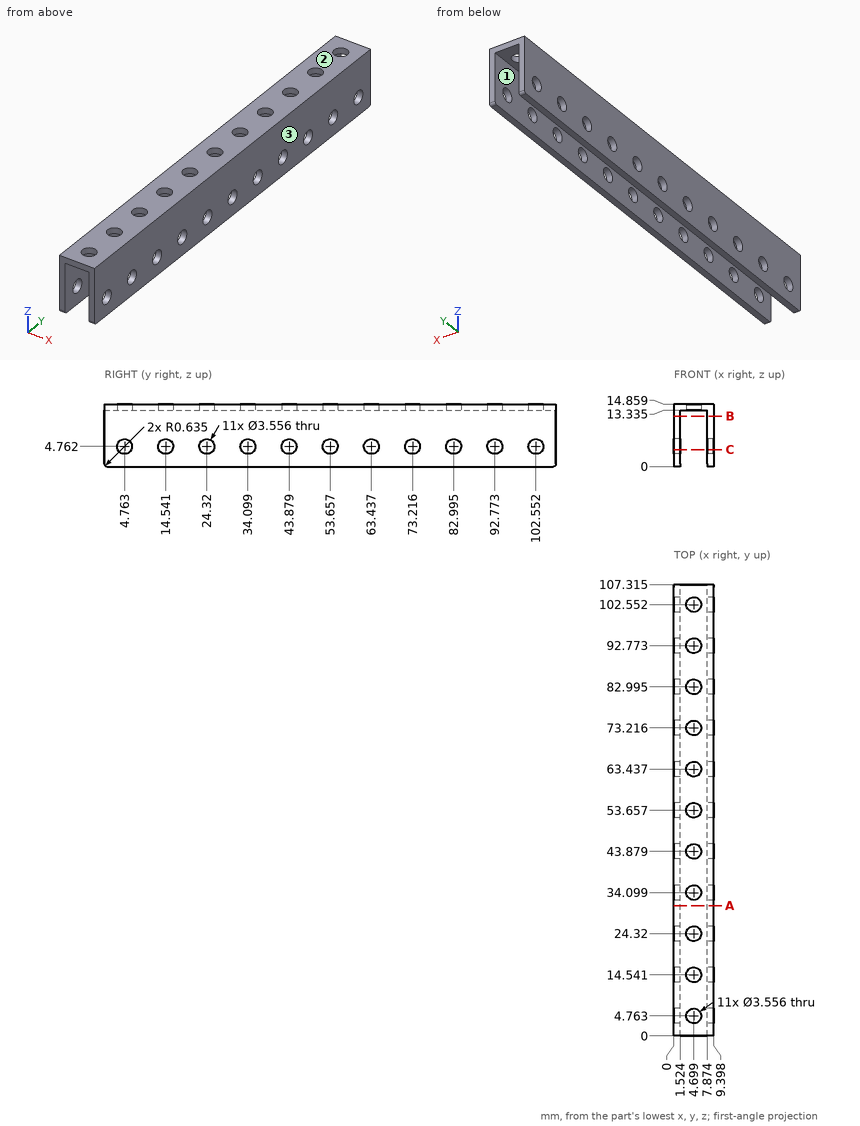
Here's the drawing with two shaded views (mm, measured from the low corner). I have some questions. Round coordinates to 2 decimals unless told otherwise and drop trailing zeros. Order: outer loops, then holes, each group sorted by start corner. A loop starts at its lowest first (then second) coordinate and runs counter-clockwise, first axis right, second up. Notation, with made-up numbers: M -6.5,68 L -2.5,68 A28 cw -2.5,98 Z; hole C 19.25,73 d6. An arc over 180 degrees is marked long. Answer in a Markdown table with one row per item.
Item 1: Imagine slicing it at A-A, the plane y = 31. Write out the boundary of the cut face in (x, z) (1 decimal).
A:
| item | result |
|---|---|
| outline | M 0,0 L 1.5,0 L 1.5,13.3 L 7.9,13.3 L 7.9,0 L 9.4,0 L 9.4,14.9 L 0,14.9 Z |
Item 2: Thinking about a two-plate mould opening in X: for the marked faces 1, 2 and 3, which applies, +X half, -X half, draft (parallel to the pull), parting line (faces both ways), or undercut?
A:
| item | result |
|---|---|
| face 1 | undercut |
| face 2 | draft |
| face 3 | +X half |
Item 3: Imagine slicing it at B-B, the plane z = 12. Write out the boundary of the cut face in (x, y) (1 decimal).
A:
| item | result |
|---|---|
| outline | M 0,0 L 1.5,0 L 1.5,107.3 L 0,107.3 Z; M 7.9,0 L 9.4,0 L 9.4,107.3 L 7.9,107.3 Z |
Item 4: Imagine slicing it at C-C, the plane z = 4. State how many separate pieces and enclosed holes the cut face has.
A:
| item | result |
|---|---|
| separate pieces | 24 |
| enclosed holes | 0 |
Item 5: I'm going to push flat-ended pins straight in: pin 1 (2 mm diameter, centred on x = 4.7, y = 73.22, fed in from +Z); pin 2 (4 mm diameter, centred on x = 4.7, y = 53.66, fed in from -Z) (1 decimal). Where does each tip first touch, or does it pass through?
A:
| item | result |
|---|---|
| pin 1 | passes through |
| pin 2 | stops at z = 13.3 |
Item 6: If I drill on L1, parallel to X at y = 95.5, z = 6 (1 decimal); L2, parallel to Z at x = 6.25, y = 62 (1 decimal), over which ranges is the centre line in solid material (lowest first)? Write a range as from..to.
A:
| item | result |
|---|---|
| L1 | x = 0..1.5, 7.9..9.4 |
| L2 | z = 13.3..14.9 |
